The model under review builds one solid part; all positions refer to its coordinate system, in mm. A direction names the side the tool comes from. Round coordinates to 2 decimals unless told otherwise and drop trailing zeros. Loops run counter-clockwise (first coordinate to the right, second up) from the corner with the lowest first, then second, coordinate; pieces in that order, holes last. Notation, with made-up numbers: M -4,42 L 24,42 A18 ccw 24,75 Z; hole C 89.25,2 d2. An arc over 180 degrees is marked long. Return JSON: item names as keys, results as strings. Group by question number.
Q1. Consider section D-D (y = 123). State the section outline as (x, z) points, and give its area (3 significant figures).
Q2. To check wall thickness, follow line 1 along X through (y, z) = (399.5, 1); line 2 along Y through (x, z) = (210.5, 10); line 3 along X through (y, z) = (105, 2). State the ranges of each line that lie inside material, in increasing order.
Q3. Consider section B-B (y = 490). State the section outline as (x, z) points, and give its area (3 significant figures).
Q4. Clearance check with flat-ended pins moving along their axes: pin 1 Ø6 at (x, z) = (303, 3) entering from -Y; pin 2 Ø5 at (x, y) = (48.64, 107.72) entering from +Z. State where each tip first meets the part, or that it passes through.
Q5. Consider section C-C (z = 8). Count the separate pieces of the cut face and the enclosed holes in it, and give its area (3 significant figures).
Q6. Consider section A-A (x = 172.85). State the section outline as (y, z) points.
Q7. Draft analysis for pull direction X (two halves, no side actions). For faces 1 (the face through (170, 337, 18)), 2 (the face through (0, 268, 9)), 3 (the face through (317.61, 369.69, 9.13)), 4 (the face through (27.69, 370.09, 9.13)), state which applies: pulls with the +X half, pulls with the -X half, needs draft (parallel to the pull), parting line crosses it, or undercut.
Q8. For faces 5 (the face through (170, 337, 0)), 6 (the face through (171, 362.45, 9)), list the 3-axis set-ups (+Z, -Z, +X, -X, +Y, -Y) from which the entire face can be reached by the end or side of a thin tool; tool diameter is ignored.
from build123d import *

# Parameters (mm, degrees)
SKETCH1_W           = 345.7
SKETCH1_H           = 544.6
BOSS_EXTRUDE1_DEPTH = 18
SKETCH2_W           = 266.7
SKETCH2_H           = 127
CUT_EXTRUDE1_DEPTH  = 19
SKETCH3_R           = 139.065
CUT_EXTRUDE2_DEPTH  = 19
SKETCH4_R           = 3.175
CUT_EXTRUDE3_DEPTH  = 19
CUT_EXTRUDE4_DEPTH  = 19


with BuildPart() as part:
    # Sketch1 → Boss-Extrude1 (new body)
    with BuildSketch(Plane.XY):
        with Locations((172.85, 272.3)):
            Rectangle(SKETCH1_W, SKETCH1_H)
    extrude(amount=BOSS_EXTRUDE1_DEPTH)

    # Sketch2 → Cut-Extrude1 (cut, through all)
    with BuildSketch(Plane.XY.offset(18)):
        with Locations((172.85, 445)):
            Rectangle(SKETCH2_W, SKETCH2_H)
    extrude(amount=-CUT_EXTRUDE1_DEPTH, mode=Mode.SUBTRACT)

    # Sketch3 → Cut-Extrude2 (cut, through all)
    with BuildSketch(Plane.XY.offset(18)):
        with Locations((172.85, 186.690965799)):
            Circle(SKETCH3_R)
    extrude(amount=-CUT_EXTRUDE2_DEPTH, mode=Mode.SUBTRACT)

    # Sketch4 → Cut-Extrude3 (cut, through all)
    with BuildSketch(Plane.XY.offset(18)):
        with Locations((204.842157428, 330.365184475)):
            Circle(SKETCH4_R)
        with Locations((297.06488577, 265.662108644)):
            Circle(SKETCH4_R)
        with Locations((316.524218676, 154.698808371)):
            Circle(SKETCH4_R)
        with Locations((251.821142845, 62.476080029)):
            Circle(SKETCH4_R)
        with Locations((140.857842572, 43.016747123)):
            Circle(SKETCH4_R)
        with Locations((48.63511423, 107.719822954)):
            Circle(SKETCH4_R)
        with Locations((29.175781324, 218.683123227)):
            Circle(SKETCH4_R)
        with Locations((93.878857155, 310.905851569)):
            Circle(SKETCH4_R)
    extrude(amount=-CUT_EXTRUDE3_DEPTH, mode=Mode.SUBTRACT)

    # Sketch6 → Cut-Extrude4 (cut, through all)
    with BuildSketch(Plane.XY.offset(18)):
        with BuildLine():
            Line((45.85, 362.45), (299.85, 362.45))
            ThreePointArc((299.85, 362.45), (317.810512242, 369.889487758), (325.25, 387.85))
            Line((325.25, 387.85), (325.25, 502.15))
            ThreePointArc((325.25, 502.15), (317.810512242, 520.110512242), (299.85, 527.55))
            Line((299.85, 527.55), (45.85, 527.55))
            ThreePointArc((45.85, 527.55), (27.889487758, 520.110512242), (20.45, 502.15))
            Line((20.45, 502.15), (20.45, 387.85))
            ThreePointArc((20.45, 387.85), (27.889487758, 369.889487758), (45.85, 362.45))
        make_face()
    extrude(amount=-CUT_EXTRUDE4_DEPTH, mode=Mode.SUBTRACT)


solid = part.part
Values:
{
 "1": {"outline": "M 0,0 L 49.23,0 L 49.23,18 L 0,18 Z; M 296.47,0 L 345.7,0 L 345.7,18 L 296.47,18 Z", "area": "1,770 mm2"},
 "2": {"line 1": "x = 0 to 20.45, 325.25 to 345.7", "line 2": "y = 0 to 52.82, 320.56 to 362.45, 527.55 to 544.6", "line 3": "x = 0 to 47, 50.27 to 60.31, 285.39 to 345.7"},
 "3": {"outline": "M 0,0 L 20.45,0 L 20.45,18 L 0,18 Z; M 325.25,0 L 345.7,0 L 345.7,18 L 325.25,18 Z", "area": "736 mm2"},
 "4": {"pin 1": "stops at y = 0", "pin 2": "passes through"},
 "5": {"separate pieces": "1", "enclosed holes": "10", "area": "77,500 mm2"},
 "6": {"outline": "M 0,0 L 47.63,0 L 47.63,18 L 0,18 Z; M 325.76,0 L 362.45,0 L 362.45,18 L 325.76,18 Z; M 527.55,0 L 544.6,0 L 544.6,18 L 527.55,18 Z"},
 "7": {"face 1": "needs draft", "face 2": "pulls with the -X half", "face 3": "undercut", "face 4": "undercut"},
 "8": {"face 5": "-Z, +X, -X, +Y, -Y", "face 6": "+Z, -Z"}
}
